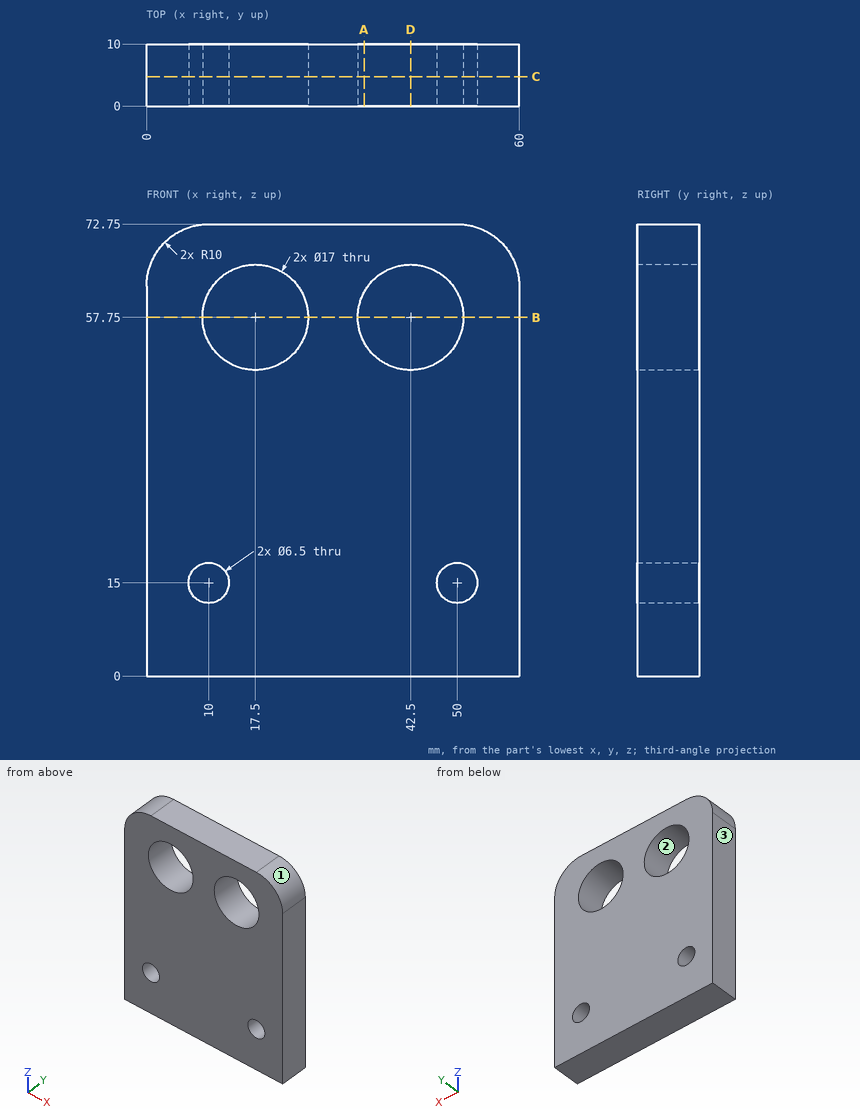
For this review, use the dimensioned drawing (mm, ordinates from the lowest corner) and the shaded views. Coordinates: 2 decimals unless noted, no trailing zeros. Loops run counter-clockwise (first coordinate to the right, second up) from the corner with the lowest first, then second, coordinate; pieces in that order, holes last. Notation, with made-up numbers: (10.5, 48) - (69.5, 48) arc R21 cw to (69.5, 70) - close; hole circle Ø9 at (83.5, 65.5). An arc over 180 degrees is marked (long way). Use one line per item in the form item = value. Start each with the question number.
1) To check wall thickness, follow probe 1 along X at (y, z) = (6, 15); probe 2 along X at (y, z) = (5, 65); probe 3 along Z at (x, y) = (18, 6.75). State the ranges of each line that lie inside material, in increasing order. Write a range as from..to.
2) Take a section at D-D (x = 42.5). State the section outline as (y, z) points, plus the area to 4 significant figures.
3) Take a section at B-B (z = 57.75). State the section outline as (x, y) points, plus the area to 3 significant figures.
4) Take a section at A-A (x = 35). State the section outline as (y, z) points, plus the area to 4 significant figures.
5) Draft analysis for pull direction X (two halves, no side actions). For the marked faces 1, 2 and 3, state which applies: released by +X, released by -X, zero draft, split by the parting line, or undercut.
6) Take a section at C-C (y = 4.75). State the section outline as (x, z) points, plus the area to 3 significant figures.
From the geometry:
q1.probe_1 = 0..6.75, 13.25..46.75, 53.25..60
q1.probe_2 = 0.26..13.06, 21.94..38.06, 46.94..59.74
q1.probe_3 = 0..49.26, 66.24..72.75
q2.outline = (0, 0) - (10, 0) - (10, 49.25) - (0, 49.25) - close; (0, 66.25) - (10, 66.25) - (10, 72.75) - (0, 72.75) - close
q2.area = 557.5 mm2
q3.outline = (0, 0) - (9, 0) - (9, 10) - (0, 10) - close; (26, 0) - (34, 0) - (34, 10) - (26, 10) - close; (51, 0) - (60, 0) - (60, 10) - (51, 10) - close
q3.area = 260 mm2
q4.outline = (0, 0) - (10, 0) - (10, 53.75) - (0, 53.75) - close; (0, 61.75) - (10, 61.75) - (10, 72.75) - (0, 72.75) - close
q4.area = 647.5 mm2
q5.face_1 = released by +X
q5.face_2 = undercut
q5.face_3 = released by -X
q6.outline = (0, 0) - (60, 0) - (60, 62.75) arc R10 ccw to (50, 72.75) - (10, 72.75) arc R10 ccw to (0, 62.75) - close; hole circle Ø6.5 at (10, 15); hole circle Ø17 at (17.5, 57.75); hole circle Ø17 at (42.5, 57.75); hole circle Ø6.5 at (50, 15)
q6.area = 3,800 mm2
